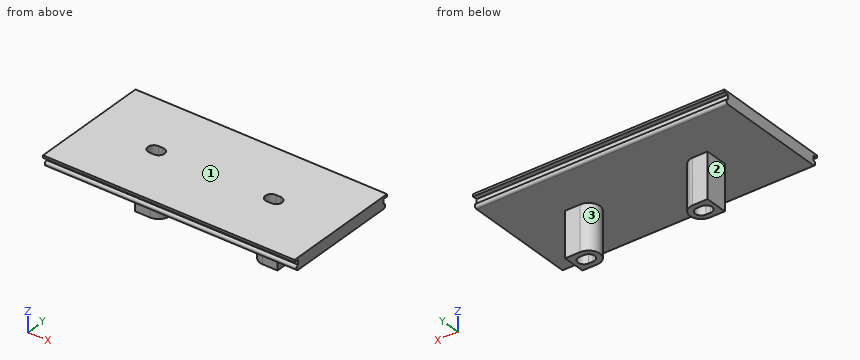
from build123d import *

# Parameters (mm, degrees)
F0_W     = 106
F0_H     = 47
F1_DEPTH = 2
F3_DEPTH = 1
F5_DEPTH = 106
F7_DEPTH = 19
F8_DEPTH = 25


with BuildPart() as f1:
    # F0 (on Top) → F1 (new body)
    with BuildSketch(Plane.XY):
        with Locations((53, 23.5)):
            Rectangle(F0_W, F0_H)
    extrude(amount=F1_DEPTH)

    # F2 (on face) → F3 (join)
    with BuildSketch(Plane.XY.offset(2)):
        Polygon((0, 49), (0, 0), (0, -2), (106, -2), (106, 49), align=None)
    extrude(amount=F3_DEPTH)

    # F4 (on face) → F5 (join)
    with BuildSketch(Plane.YZ.offset(106)):
        with BuildLine():
            Line((47, 0), (0, 0))
            ThreePointArc((0, 0), (-1, -1), (0, -2))
            Line((0, -2), (47, -2))
            ThreePointArc((47, -2), (48, -1), (47, 0))
        make_face()
    extrude(amount=-F5_DEPTH)

    # F6 (on face) → F7 (join)
    with BuildSketch(Plane(origin=(0, 0, -2), x_dir=(1, 0, 0), z_dir=(0, 0, -1))):
        with BuildLine():
            Line((23, -28.25), (29.25, -28.25))
            ThreePointArc((29.25, -28.25), (34, -23.5), (29.25, -18.75))
            Line((29.25, -18.75), (23, -18.75))
            Line((23, -18.75), (23, -28.25))
        make_face()
        with BuildLine():
            Line((27.25, -21), (29.25, -21))
            ThreePointArc((29.25, -21), (31.75, -23.5), (29.25, -26))
            Line((29.25, -26), (27.25, -26))
            ThreePointArc((27.25, -26), (24.75, -23.5), (27.25, -21))
        make_face(mode=Mode.SUBTRACT)
        with BuildLine():
            Line((83, -18.75), (76.75, -18.75))
            ThreePointArc((76.75, -18.75), (72, -23.5), (76.75, -28.25))
            Line((76.75, -28.25), (83, -28.25))
            Line((83, -28.25), (83, -18.75))
        make_face()
        with BuildLine():
            ThreePointArc((76.75, -26), (74.25, -23.5), (76.75, -21))
            Line((76.75, -21), (78.75, -21))
            ThreePointArc((78.75, -21), (81.25, -23.5), (78.75, -26))
            Line((78.75, -26), (76.75, -26))
        make_face(mode=Mode.SUBTRACT)
    extrude(amount=F7_DEPTH)

    # F8 (cut): faces of the model
    f8_faces = [f1.faces().sort_by_distance(p)[0] for p in [
        (28.25, 23.5, -2),
        (77.75, 23.5, -2),
    ]]
    extrude(f8_faces, amount=-F8_DEPTH, mode=Mode.SUBTRACT)


solid = f1.part
CAD build for the part. Positions are in the model's coordinates, mm. Face numbers are marked on the shaded views. Give positions to 0.01 mm unless a question says otherwise; leave off trailing zeros. Order: outer loops, then holes, each group sorted by start corner. A loop starts at its lowest first (then second) coordinate and runs counter-clockwise, first axis right, second up. Notation, with made-up numbers: (15, -37.75) - (43, -37.75) arc R19 ccw to (43, -15.75) - close; hole circle Ø5 at (-5.75, 83). An arc over 180 degrees is marked (long way). Answer in a Markdown table with one row per item.
1. Saw through at D-D, the plane x = 93. Give the cut face in (y, z), plus the area to 3 significant figures.
Data:
| item | result |
|---|---|
| outline | (-2, 2) - (0, 2) - (0, 0) arc R1 ccw to (0, -2) - (47, -2) arc R1 ccw to (47, 0) - (47, 2) - (49, 2) - (49, 3) - (-2, 3) - close |
| area | 242 mm² |
2. Saw through at B-B, the plane y = 23.5. Give the cut face in (x, z).
Data:
| item | result |
|---|---|
| outline | (0, -2) - (23, -2) - (23, -21) - (24.75, -21) - (24.75, 3) - (0, 3) - close; (31.75, -21) - (34, -21) - (34, -2) - (72, -2) - (72, -21) - (74.25, -21) - (74.25, 3) - (31.75, 3) - close; (81.25, -21) - (83, -21) - (83, -2) - (106, -2) - (106, 3) - (81.25, 3) - close |
3. Pull direction X, two halves, no side cores. Call the marked faces 1, 2 and 3: pulls with the +X half, pulls with the -X half, needs draft (parallel to the pull), parting line crosses it, or undercut.
Data:
| item | result |
|---|---|
| face 1 | needs draft |
| face 2 | pulls with the -X half |
| face 3 | undercut |
4. Saw through at A-A, the plane z = -3.25. Give the cut face in (x, y).
Data:
| item | result |
|---|---|
| outline | (23, 18.75) - (29.25, 18.75) arc R4.75 ccw to (29.25, 28.25) - (23, 28.25) - close; (76.75, 18.75) - (83, 18.75) - (83, 28.25) - (76.75, 28.25) arc R4.75 ccw to start; hole (27.25, 21) - (29.25, 21) arc R2.5 ccw to (29.25, 26) - (27.25, 26) arc R2.5 ccw to start; hole (76.75, 21) - (78.75, 21) arc R2.5 ccw to (78.75, 26) - (76.75, 26) arc R2.5 ccw to start |
5. Flat gauge pins, fed straight in: pin 1 (1.6 mm diameter, centred on x = 28.5, z = -14.5, fed in from -Y); pin 2 (0.6 mm diameter, centred on x = 49.5, y = -1, fed in from -Z); pin 3 (4 mm diameter, centred on y = 30, z = -4.5, fed in from -X). Where does each tip first touch, or does it go through?
Data:
| item | result |
|---|---|
| pin 1 | stops at y = 18.75 |
| pin 2 | stops at z = -1.71 |
| pin 3 | stops at x = 23 |
6. Probe probe 1 along Y at (x, z) = (27, -17.75); probe 2 along Z at (x, y) = (32, 3); probe 3 along Y at (x, z) = (7.5, -1). List the from-to ranges inside material, lowest first. Write a range as [from, to].
Data:
| item | result |
|---|---|
| probe 1 | y = [18.75, 21.01], [25.99, 28.25] |
| probe 2 | z = [-2, 3] |
| probe 3 | y = [-1, 48] |
7. Saw through at C-C, the plane z = 1. Give the cut face in (x, y).
Data:
| item | result |
|---|---|
| outline | (0, 0) - (106, 0) - (106, 47) - (0, 47) - close; hole (27.25, 21) - (29.25, 21) arc R2.5 ccw to (29.25, 26) - (27.25, 26) arc R2.5 ccw to start; hole (76.75, 21) - (78.75, 21) arc R2.5 ccw to (78.75, 26) - (76.75, 26) arc R2.5 ccw to start |
